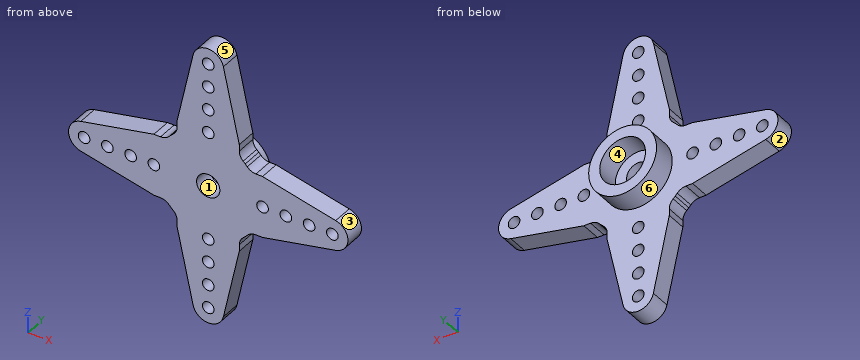
```python
from build123d import *

# Parameters (mm, degrees)
CROQUIS1_R              = 0.75
CROQUIS1_R_2            = 1.5
SALIENTE_EXTRUIR1_DEPTH = 2.6
CROQUIS2_R              = 4.375
CROQUIS2_R_2            = 2.95
SALIENTE_EXTRUIR2_DEPTH = 3


with BuildPart() as part:
    # Croquis1 → Saliente-Extruir1 (new body)
    with BuildSketch(Plane(origin=(0, 0, 0), x_dir=(1, 0, 0), z_dir=(0, 1, 0))):
        with BuildLine():
            Line((-4, 7), (-4, 6.149186938))
            ThreePointArc((-4, 6.149186938), (-4.130693606, 5.536814502), (-4.5, 5.031152949))
            ThreePointArc((-4.5, 5.031152949), (-4.638282144, 4.903961537), (-4.772970773, 4.772970773))
            ThreePointArc((-4.772970773, 4.772970773), (-4.903961537, 4.638282144), (-5.031152949, 4.5))
            ThreePointArc((-5.031152949, 4.5), (-5.536814502, 4.130693606), (-6.149186938, 4))
            Line((-6.149186938, 4), (-7, 4))
            Line((-7, 4), (-16.424218619, 1.954491894))
            ThreePointArc((-16.424218619, 1.954491894), (-18, 0), (-16.424218619, -1.954491894))
            Line((-16.424218619, -1.954491894), (-7, -4))
            Line((-7, -4), (-6.149186938, -4))
            ThreePointArc((-6.149186938, -4), (-5.536814502, -4.130693606), (-5.031152949, -4.5))
            ThreePointArc((-5.031152949, -4.5), (-4.903961537, -4.638282144), (-4.772970773, -4.772970773))
            ThreePointArc((-4.772970773, -4.772970773), (-4.638282144, -4.903961537), (-4.5, -5.031152949))
            ThreePointArc((-4.5, -5.031152949), (-4.130693606, -5.536814502), (-4, -6.149186938))
            Line((-4, -6.149186938), (-4, -7))
            Line((-4, -7), (-1.954491894, -16.424218619))
            ThreePointArc((-1.954491894, -16.424218619), (0, -18), (1.954491894, -16.424218619))
            Line((1.954491894, -16.424218619), (4, -7))
            Line((4, -7), (4, -6.149186938))
            ThreePointArc((4, -6.149186938), (4.130693606, -5.536814502), (4.5, -5.031152949))
            ThreePointArc((4.5, -5.031152949), (4.638282144, -4.903961537), (4.772970773, -4.772970773))
            ThreePointArc((4.772970773, -4.772970773), (4.903961537, -4.638282144), (5.031152949, -4.5))
            ThreePointArc((5.031152949, -4.5), (5.536814502, -4.130693606), (6.149186938, -4))
            Line((6.149186938, -4), (7, -4))
            Line((7, -4), (16.424218619, -1.954491894))
            ThreePointArc((16.424218619, -1.954491894), (18, 0), (16.424218619, 1.954491894))
            Line((16.424218619, 1.954491894), (7, 4))
            Line((7, 4), (6.149186938, 4))
            ThreePointArc((6.149186938, 4), (5.536814502, 4.130693606), (5.031152949, 4.5))
            ThreePointArc((5.031152949, 4.5), (4.903961537, 4.638282144), (4.772970773, 4.772970773))
            ThreePointArc((4.772970773, 4.772970773), (4.638282144, 4.903961537), (4.5, 5.031152949))
            ThreePointArc((4.5, 5.031152949), (4.130693606, 5.536814502), (4, 6.149186938))
            Line((4, 6.149186938), (4, 7))
            Line((4, 7), (1.954491894, 16.424218619))
            ThreePointArc((1.954491894, 16.424218619), (0, 18), (-1.954491894, 16.424218619))
            Line((-1.954491894, 16.424218619), (-4, 7))
        make_face()
        with Locations(Location((0, 16, 0), (0, 0, 270))):
            Circle(CROQUIS1_R, mode=Mode.SUBTRACT)
        with Locations(Location((0, 13, 0), (0, 0, 270))):
            Circle(CROQUIS1_R, mode=Mode.SUBTRACT)
        with Locations(Location((0, 10, 0), (0, 0, 270))):
            Circle(CROQUIS1_R, mode=Mode.SUBTRACT)
        with Locations(Location((0, 7, 0), (0, 0, 270))):
            Circle(CROQUIS1_R, mode=Mode.SUBTRACT)
        with Locations(Location((16, 0, 0), (0, 0, 270))):
            Circle(CROQUIS1_R, mode=Mode.SUBTRACT)
        with Locations(Location((13, 0, 0), (0, 0, 270))):
            Circle(CROQUIS1_R, mode=Mode.SUBTRACT)
        with Locations(Location((10, 0, 0), (0, 0, 270))):
            Circle(CROQUIS1_R, mode=Mode.SUBTRACT)
        with Locations(Location((7, 0, 0), (0, 0, 270))):
            Circle(CROQUIS1_R, mode=Mode.SUBTRACT)
        with Locations(Location((0, -16, 0), (0, 0, 270))):
            Circle(CROQUIS1_R, mode=Mode.SUBTRACT)
        with Locations(Location((0, -13, 0), (0, 0, 270))):
            Circle(CROQUIS1_R, mode=Mode.SUBTRACT)
        with Locations(Location((0, -10, 0), (0, 0, 270))):
            Circle(CROQUIS1_R, mode=Mode.SUBTRACT)
        with Locations(Location((0, -7, 0), (0, 0, 270))):
            Circle(CROQUIS1_R, mode=Mode.SUBTRACT)
        with Locations(Location((-16, 0, 0), (0, 0, 270))):
            Circle(CROQUIS1_R, mode=Mode.SUBTRACT)
        with Locations(Location((-13, 0, 0), (0, 0, 270))):
            Circle(CROQUIS1_R, mode=Mode.SUBTRACT)
        with Locations(Location((-10, 0, 0), (0, 0, 270))):
            Circle(CROQUIS1_R, mode=Mode.SUBTRACT)
        with Locations(Location((-7, 0, 0), (0, 0, 270))):
            Circle(CROQUIS1_R, mode=Mode.SUBTRACT)
        with Locations(Location((0, 0, 0), (0, 0, 270))):
            Circle(CROQUIS1_R_2, mode=Mode.SUBTRACT)
    extrude(amount=SALIENTE_EXTRUIR1_DEPTH)

    # Croquis2 → Saliente-Extruir2 (add)
    with BuildSketch(Plane(origin=(0, 2.6, 0), x_dir=(1, 0, 0), z_dir=(0, 1, 0))):
        with Locations(Location((0, 0, 0), (0, 0, 270))):
            Circle(CROQUIS2_R)
        with Locations(Location((0, 0, 0), (0, 0, 270))):
            Circle(CROQUIS2_R_2, mode=Mode.SUBTRACT)
    extrude(amount=SALIENTE_EXTRUIR2_DEPTH)


solid = part.part
```
The model under review builds one solid part; all positions refer to its coordinate system, in mm. Face numbers are marked on the shaded views. A direction names the side the tool comes from. Round coordinates to 2 decimals unless told otherwise and drop trailing zeros. Write each loop counter-clockwise with the first axis right and the second up, starting at its lowest first coordinate (ties: lowest second). Pieces come first, ordered by that corner, then holes. Notation, with made-up numbers: M 89.5,49 L 135.5,49 A18 ccw 135.5,78 Z; hole C 48,84 d6. An arc over 180 degrees is marked long. Use CSV: the item, a comma, the result in double quotes. Start each with the question number.
(1) The part is to be moulded in two halves that separate along X. For the marked faces 1, 2, 3 and 4, say which applies: +X half, -X half, draft (parallel to the pull), parting line (faces both ways), or undercut.
(2) For line 1 along Z through (x, y) = (-2.5, 3.3); line 2 along Y through (x, z) = (-3, 6); line 3 along X through (y, z) = (4, 1.5), list the stretches that pass through material, from the lowest coordinate up.
(3) We need section D-D, the plane x = 0. State how many separate pieces and enclosed holes the cut face has, then the cut area to 4 significant figures.
(4) We need section C-C, the plane y = 5. State the section outline as (x, z) points (3 decimals).
(5) Clearance check with flat-ended pins moving along their axes: P1, Ø2, axis at x = -10, z = 0, coming from the +Y side; P2, Ø0.7, axis at x = -6.5, y = 1, coming from the +Z side; P3, Ø0.9, axis at y = 1.5, z = 6.5, coming from the -X side. State where each tip first meets the part, or that it passes through.
(6) Tool access review of the marked faces 5 and 6: name each direction out of +Z, -Z, +X, -X, +Y, -Y from which nothing blocks a thin tool from reaching the whole face with its end or side.
(7) We need section A-A, the plane z = -13. State the section outline as (x, y) points, then the cut area to 3 significant figures.
(8) We need section B-B, the plane x = -16. State the section outline as (y, z) points, then the cut area to 3 significant figures.
Findings:
1,face 1,"undercut"
1,face 2,"-X half"
1,face 3,"+X half"
1,face 4,"undercut"
2,line 1,"-3.59 to -1.57, 1.57 to 3.59"
2,line 2,"0 to 2.6"
2,line 3,"-4.11 to -2.54, 2.54 to 4.11"
3,separate pieces,"10"
3,enclosed holes,"0"
3,area,"63.15 mm^2"
4,outline,"C 0,0 d8.75; hole C 0,0 d5.9"
5,P1,"y = 2.6"
5,P2,"z = 4"
5,P3,"x = -4"
6,face 5,"+Z, +Y, -Y"
6,face 6,"+Y"
7,outline,"M -2.7,0 L -0.75,0 L -0.75,2.6 L -2.7,2.6 Z; M 0.75,0 L 2.7,0 L 2.7,2.6 L 0.75,2.6 Z"
7,area,"10.1 mm^2"
8,outline,"M 0,-2.05 L 2.6,-2.05 L 2.6,-0.75 L 0,-0.75 Z; M 0,0.75 L 2.6,0.75 L 2.6,2.05 L 0,2.05 Z"
8,area,"6.74 mm^2"
